Check sheet for the modelled part. Datum: model origin and axes. Units: mm. A direction names the side the tool comes from. Coordinates: 2 decimals unless noted, no trailing zeros. Loops run counter-clockwise (first coordinate to the right, second up) from the corner with the lowest first, then second, coordinate; pieces in that order, holes last. Notation, with made-up numbers: M -28.5,51.25 L -5.5,51.25 A26 cw -5.5,81.25 Z; hole C 6.25,10 d9. An arc over 180 degrees is marked long. Write each question's results on one line, items separated by ' | '. Start each with the question number.
Autodesk Inventor part; units mm, degrees
ref_plane "YZ Plane" through (0, 0, 0) normal (1, 0, 0) x (0, 1, 0)
ref_plane "XZ Plane" through (0, 0, 0) normal (0, 1, 0) x (-1, 0, 0)
ref_plane "XY Plane" through (0, 0, 0) normal (0, 0, 1) x (1, 0, 0)
sketch "Boceto5" plane through (0, 0, 0) normal (0, 1, 0) x (-1, 0, 0)
  line L0 (10.2966, 28.3637) -> (10.2966, 8.3637)
  line L1 (10.2966, 8.3637) -> (-169.7034, 8.3637)
  line L2 (-169.7034, 8.3637) -> (-169.7034, 28.3637)
  line L3 (-169.7034, 28.3637) -> (10.2966, 28.3637)
  line L4 (10.2966, 18.3637) -> (-169.7034, 18.3637)
  circle A0 centre (-154.7034, 23.3637) radius 3
  circle A1 centre (-4.7034, 23.3637) radius 3
  circle A2 centre (-14.7034, 13.3637) radius 3
  circle A3 centre (-144.7034, 13.3637) radius 3
  circle A4 centre (-72.7034, 23.3637) radius 2
  point P0 (0, 0)
  dimension "d33" = 20
  dimension "d34" = 180
  dimension "d35" = 20
  dimension "d36" = 6
  dimension "d37" = 6
  dimension "d38" = 6
  dimension "d39" = 6
  dimension "d40" = 150
  dimension "d41" = 130
  dimension "d42" = 15
  dimension "d43" = 25
  dimension "d44" = 5
  dimension "d45" = 5
  dimension "d46" = 5
  dimension "d47" = 5
  dimension "d54" = 4
  dimension "d56" = 5
  dimension "d57" = 83
extrude "Extrusión4" add sketch "Boceto5" along normal blind 2 contours L0 L1 L2 L4
extrude "Extrusión5" add sketch "Boceto5" along normal blind 2 contours L0 L4 L2 L3
bend part "Pieza de plegado1" radius 0.5 angle 90 line through (-10.2966, 0, 18.3637) along (1, 0, 0) centre toward (0, -1, 0) moving side (0, 0, -1) both sides no
equation "\"Radio_pliegue\" = Grosor"
equation "\"Anchura_desahogo_plegado\" = Grosor"
equation "\"Profundidad_desahogo_plegado\" = 0.5 * Grosor"
equation "\"Tamaño_destalonado\" = 4 * Grosor"
equation "\"Remanente_mínimo\" = 2 * Grosor"
equation "\"Radiodetransición\" = Radio_pliegue"
equation "\"Tamaño_de_radio_de_Jacobi\" = Grosor"
equation "\"TamañoSeparación\" = Grosor"
properties part number "Soporte en L Frontal" material "Aluminum 1100-H14"
Item 1: Release check for a two-part mould opening along Z. For faces 1 (the face through (157.7, 1, 23.2)), 2 (the face through (17.7, -4.85, 16.88)), 3 (the face through (81, -5, 15.864)) record: +Z half, -Z half, draft (parallel to the pull), parting line (faces both ways), or undercut.
Item 2: Section check B-B (x = 155). Record the cut outline in (y, z), plus the area to 3 significant figures.
Item 3: Depth check by flat-ended pin: P1, Ø3, axis at x = 70, y = -4.5, coming from the +Z side; P2, Ø2, axis at x = 77.5, z = 22.5, coming from the -Y side. Enter the tip coordinate at first touch or a pass-through.
Item 4: Tool access check on faces 4 (the face through (6.915, 0.986, 21.336)), 5 (the face through (81, -5, 17.864)). Record the directions out of +Z, -Z, +X, -X, +Y, -Y that give a thin tool (end or side, any length) a straight path to the whole face; none if there is none.
Item 5: Section check A-A (x = 22). Record the cut outline in (y, z).
Item 6: Thickness scan on line 1 (X direction, y = -4.5, z = 17); line 2 (X direction, y = -7, z = 17.5); line 3 (Y direction, x = 41, z = 21.75). Record the ranges inside material, lowest first.
Computed values:
1) face 1: undercut | face 2: draft | face 3: -Z half
2) outline: M -9.71,15.86 L -0.5,15.86 A2.5 ccw 2,18.36 L 2,20.38 L 0,20.38 L 0,18.36 A0.5 cw -0.5,17.86 L -9.71,17.86 Z; M 0,26.35 L 2,26.35 L 2,28.36 L 0,28.36 Z | area: 31.2 mm²
3) P1: stops at z = 17.86 | P2: stops at y = 0
4) face 4: +Y, -Y | face 5: +Z, +X, -X, -Y
5) outline: M -9.71,15.86 L -0.5,15.86 A2.5 ccw 2,18.36 L 2,28.36 L 0,28.36 L 0,18.36 A0.5 cw -0.5,17.86 L -9.71,17.86 Z
6) line 1: x = -10.3 to 11.71, 17.7 to 141.71, 147.7 to 169.7 | line 2: x = -10.3 to 12.76, 16.65 to 142.76, 146.65 to 169.7 | line 3: y = 0 to 2
